Work out the finished part from the listing and answer in its coordinate system (mm). A direction names the side the tool comes from. Give positions to 0.01 mm unless a question says otherwise; leave off trailing zeros. Order: outer loops, then holes, each group sorted by start corner. A loop starts at its lowest first (then second) coordinate and runs counter-clockwise, first axis right, second up. Notation, with made-up numbers: (64, -20) - (108, -20) arc R16 ccw to (108, -15) - close; hole circle Ø6 at (79.5, -23). An arc over 180 degrees is marked (long way). Write each question's results on one line, items separated by ' | '.
from build123d import *

# Parameters (mm, degrees)
F0_W        = 86
F0_H        = 97
F1_DEPTH    = 3
F2_W        = 68
F2_H        = 97
F3_DEPTH    = 27.5
F4_T        = 3
F4_T3_DEPTH = 103
F7_DEPTH    = 8
F9_DEPTH    = 1.5
F10_W       = 76
F10_H       = 18.5
F11_DEPTH   = 3
F13_DEPTH   = 1.1


# Not quite as in the source:
# - a shell that OpenCascade refuses in one call is made with other operations: the cavity is built on its own and cut out


with BuildPart() as f1:
    # F0 (on Top) → F1 (new body)
    with BuildSketch(Plane.XY):
        with Locations((43, 48.5)):
            Rectangle(F0_W, F0_H)
    extrude(amount=F1_DEPTH)

    # F2 (on face) → F3 (join)
    with BuildSketch(Plane.XY.offset(3)):
        with Locations((43, 48.5)):
            Rectangle(F2_W, F2_H)
    extrude(amount=F3_DEPTH)

    # F4: shell of thickness 3, made by hand


with BuildPart() as f4_core1:
    # F4_t2: copy of F1
    add(f1.part)

    # the walls: a layer under each face that stays
    f4_faces = [f4_core1.faces().sort_by_distance(p)[0] for p in [
        (43, 97, 15.25),
        (86, 48.5, 1.5),
        (0, 48.5, 1.5),
        (43, 48.5, 0),
        (81.5, 48.5, 3),
        (4.5, 48.5, 3),
        (77, 48.5, 16.75),
        (9, 48.5, 16.75),
    ]]
    thicken(f4_faces, amount=-F4_T, mode=Mode.SUBTRACT)

    # F4_s4 → F4_t3 (cut)
    with BuildSketch(Plane.XZ.offset(-100)):
        Polygon((77.03, 3.03), (77, 0), (74, 0), (74, 3), align=None)
        Polygon((8.97, 3.03), (9, 0), (12, 0), (12, 3), align=None)
    extrude(amount=F4_T3_DEPTH, mode=Mode.SUBTRACT)


with BuildPart() as f1_1:
    add(f1.part)

    # what is left inside the walls is the cavity
    f4_cavity = [f4_core1.part.solids().sort_by_distance(p)[0] for p in [
        (43, 31.333333, 3.03),
    ]]
    add(f4_cavity, mode=Mode.SUBTRACT)

    # F6 (on mid) → F7 (join, symmetric)
    with BuildSketch(Plane.YZ.offset(43)):
        with BuildLine():
            Line((94, 29), (94, 30.5))
            Line((94, 30.5), (89.5, 30.5))
            Line((89.5, 30.5), (88.086186224, 28.556006058))
            ThreePointArc((88.086186224, 28.556006058), (87.6818181818, 28.3500919068), (87.2774501397, 28.556006058))
            Line((87.2774501397, 28.556006058), (85.8636363636, 30.5))
            Line((85.8636363636, 30.5), (83.5, 30.5))
            Line((83.5, 30.5), (83.5, 29.5))
            Line((83.5, 29.5), (85.5, 29.5))
            Line((85.5, 29.5), (86.8730820975, 27.6120121159))
            ThreePointArc((86.8730820975, 27.6120121159), (87.6818181818, 27.2001838136), (88.4905542661, 27.6120121159))
            Line((88.4905542661, 27.6120121159), (89.5, 29))
            Line((89.5, 29), (94, 29))
        make_face()
    extrude(amount=F7_DEPTH, both=True)

    # F8 (on face) → F9 (join)
    with BuildSketch(Plane.XY.offset(30.5)):
        Polygon((33, 59), (33, 94), (12, 94), (12, 59), (12, 0), (16, 0), (16, 59), align=None)
        Polygon((59, 94), (53, 94), (53, 89.5), (71, 89.5), (71, 0), (74, 0), (74, 89.5), (74, 94), (71, 94), align=None)
    extrude(amount=-F9_DEPTH)

    # F10 (on face) → F11 (cut, through all)
    with BuildSketch(Plane(origin=(9, 0, 0), x_dir=(0, -1, 0), z_dir=(-1, 0, 0))):
        with Locations((-53, 15.25)):
            Rectangle(F10_W, F10_H)
    extrude(amount=-F11_DEPTH, mode=Mode.SUBTRACT)

    # F12 (on face) → F13 (cut)
    with BuildSketch(Plane(origin=(0, 0, 0), x_dir=(1, 0, 0), z_dir=(0, 0, -1))):
        Polygon((0, 0), (0, -97), (10.1, -97), (75.9, -97), (86, -97), (86, 0), (75.9, 0), (75.9, -93.9), (10.1, -93.9), (10.1, 0), align=None)
    extrude(amount=-F13_DEPTH, mode=Mode.SUBTRACT)


solid = f1_1.part
1. A cutting plane is placed at A-A, the plane y = 64. Write down the section's boundary in (x, z), then the cut area to 3 significant figures.
Answer list:
outline: (0, 1.1) - (10.1, 1.1) - (10.1, 0) - (75.9, 0) - (75.9, 1.1) - (86, 1.1) - (86, 3) - (77, 3) - (77, 30.5) - (71, 30.5) - (71, 29) - (74, 29) - (74, 3) - (12, 3) - (12, 6) - (9, 6) - (9, 3) - (0, 3) - close; (9, 24.5) - (12, 24.5) - (12, 29) - (33, 29) - (33, 30.5) - (9, 30.5) - close | area: 381 mm^2
2. Determine the mould class of faces 1 (the face through (42, 97, 16)), 2 (the face through (43, 48, 3)), 3 (the face through (43, 92, 29)), 4 (the face through (43, 0, 2)) for opening direction Y: +Y half, -Y half, draft (parallel to the pull), parting line (faces both ways), or undercut.
Answer list:
face 1: +Y half | face 2: draft | face 3: undercut | face 4: -Y half
3. A cutting plane is placed at B-B, the plane z = 8. Write down the section's boundary in (x, y).
Answer list:
outline: (9, 0) - (12, 0) - (12, 15) - (9, 15) - close; (9, 91) - (12, 91) - (12, 94) - (74, 94) - (74, 0) - (77, 0) - (77, 97) - (9, 97) - close
4. Straight lines are drawn through the part: line 1 (Z direction, x = 26, y = 59.5); line 2 (Z direction, x = 11, y = 83.5); line 3 (Y direction, x = 23.5, z = 6). For each, find the intervals that lie inside material, in ascending order. Write a range as [from, to].
Answer list:
line 1: [0, 3], [29, 30.5] | line 2: [0, 6], [24.5, 30.5] | line 3: [94, 97]
5. Given P1, Ø13, axis at y = 59.5, z = 14, coming from the +X side; P2, Ø0.8, axis at x = 23.5, z = 30, coming from the -Y side; P3, Ø0.8, axis at x = 60, z = 29.5, coming from the -Y side, each flat-ended and moving along its own axis, determine where each tip first touches the part or whether it passes through.
Answer list:
P1: x = 77 | P2: y = 59 | P3: y = 89.5
6. A cutting plane is placed at D-D, the plane y = 29.5. Write down the section's boundary in (x, z), then the cut area to 3 significant figures.
Answer list:
outline: (0, 1.1) - (10.1, 1.1) - (10.1, 0) - (75.9, 0) - (75.9, 1.1) - (86, 1.1) - (86, 3) - (77, 3) - (77, 30.5) - (71, 30.5) - (71, 29) - (74, 29) - (74, 3) - (12, 3) - (12, 6) - (9, 6) - (9, 3) - (0, 3) - close; (9, 24.5) - (12, 24.5) - (12, 29) - (16, 29) - (16, 30.5) - (9, 30.5) - close | area: 356 mm^2
7. A tool of negligible diameter and unlimited length cuts with its end or side. For faces 5 (the face through (72, 54, 29)), 6 (the face through (10, 15, 15)), 7 (the face through (77, 48, 17)), from which of +Z, -Z, +X, -X, +Y, -Y can it reach the whole face along a straight path? Write none if from no direction.
Answer list:
face 5: -Y | face 6: -X | face 7: +Z, +X, +Y, -Y
8. A cutting plane is placed at C-C, the plane x = 66.5. Write down the section's boundary in (y, z).
Answer list:
outline: (0, 0) - (93.9, 0) - (93.9, 1.1) - (97, 1.1) - (97, 30.5) - (89.5, 30.5) - (89.5, 29) - (94, 29) - (94, 3) - (0, 3) - close
